Geometry: see drawing. Coordinates: mm, zero at the bounding-box minimum. Coordinates: 2 decimals unless noted, no trailing zeros. Order: outer loops, then holes, each group sorted by start corner. A loop starts at its lowest first (then second) coordinate and runs counter-clockwise, first axis right, second up. Notation, with made-up numbers: M 38,-8 L 60,-8 A7 cw 60,-1 Z; hole C -2,-6 d10. An arc over 180 degrees is marked long. Answer in a Markdown table with one row per item.
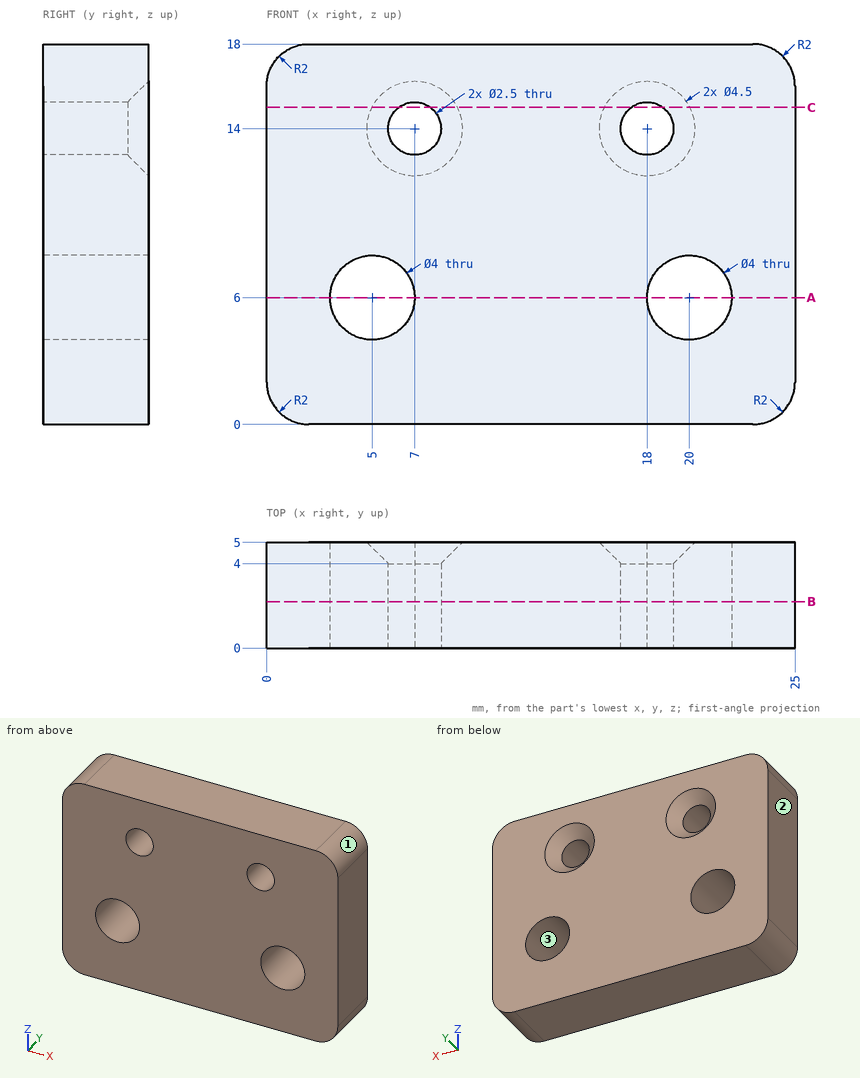
1) Cut plane B-B, the plane y = 2.2. Output: boundary loops of the cut face in (x, z).
Resolved:
| item | result |
|---|---|
| outline | M 0,2 A2 ccw 2,0 L 23,0 A2 ccw 25,2 L 25,16 A2 ccw 23,18 L 2,18 A2 ccw 0,16 Z; hole C 5,6 d4; hole C 7,14 d2.5; hole C 18,14 d2.5; hole C 20,6 d4 |
2) Cut plane A-A, the plane z = 6. Output: boundary loops of the cut face in (x, y).
Resolved:
| item | result |
|---|---|
| outline | M 0,0 L 3,0 L 3,5 L 0,5 Z; M 7,0 L 18,0 L 18,5 L 7,5 Z; M 22,0 L 25,0 L 25,5 L 22,5 Z |
3) Contact query for a flat-ended pin moving along its axis: pin 1 (3 mm diameter, centred on x = 18, z = 14, fed in from +Y). Output: stop coordinate, or through.
Resolved:
| item | result |
|---|---|
| pin 1 | stops at y = 4.25 |
4) Mould query, pull axis X, two halves, no side actions, for the marked faces 1, 2 and 3. Classes: +X half, -X half, draft (parallel to the pull), parting line (faces both ways), or undercut.
Resolved:
| item | result |
|---|---|
| face 1 | +X half |
| face 2 | -X half |
| face 3 | undercut |
5) Material intervals for probe 1 along Z at (x, y) = (5, 3.6); probe 2 along X at (y, z) = (0.95, 14.75); probe 3 along X at (y, z) = (3.75, 7.75), sorted ascending.
Resolved:
| item | result |
|---|---|
| probe 1 | z = 0 to 4, 8 to 18 |
| probe 2 | x = 0 to 6, 8 to 17, 19 to 25 |
| probe 3 | x = 0 to 4.03, 5.97 to 19.03, 20.97 to 25 |
6) Cut plane C-C, the plane z = 15. State how many separate pieces and enclosed holes the cut face has, and give its area (3 significant figures).
Resolved:
| item | result |
|---|---|
| separate pieces | 3 |
| enclosed holes | 0 |
| area | 107 mm2 |
